Geometry: final body of the model. Coordinates: model frame, mm. Face numbers are marked on the shaded views. A direction names the side the tool comes from. Round coordinates to 2 decimals unless told otherwise and drop trailing zeros. Write each loop counter-clockwise with the first axis right and the second up, starting at its lowest first coordinate (ties: lowest second). Pieces come first, ordered by that corner, then holes. Notation, with made-up numbers: M -28,-2.5 L 10,-2.5 A6 cw 10,4.5 Z; hole C 85.25,-19 d9. An arc over 180 degrees is marked long. Answer as CSV lines item,"result". Start each with the question number.
Q1. Section query C-C on x = 4. Output: boundary loops of the cut face in (y, z).
Q2. Section query D-D on z = -20. Output: boundary loops of the cut face in (x, y), and give its area (3 significant figures).
Q3. Ray query, probe 1 along Y at (x, z) = (4.5, 16); probe 2 along Z at (x, y) = (4.5, -11); probe 3 along Z at (x, y) = (5, -11). Return the intervals inside material, ascending.
Q4. Section query B-B on z = 4. Output: boundary loops of the cut face in (x, y), and give its area (3 significant figures).
Q5. First-contact query: pin 1 (2.5 mm diameter, centred on y = -11, z = 16, fed in from +X); pin 2 (12 mm diameter, centred on x = 36.5, y = 4, fed in from +Z); pin 3 (4 mm diameter, centred on x = 12.5, y = -2, fed in from -Z). Flat tips, straight axial feed; report the tip coordinate or a pass-through.
Q6. Mould query, pull axis X, two halves, no side actions, for the marked faces 4, 5 and 6. Classes: pulls with the +X half, pulls with the -X half, needs draft (parallel to the pull), parting line crosses it, or undercut.
Q7. Reachability of the marked faces 1, 2 and 3 from +Z, -Z, +X, -X, +Y, -Y: full face, straight path, thin tool, end or side. Return the list, or none.
Solid Edge part; units mm, degrees
sketch "Sketch1" plane through (0, 0, 0) normal (1, 0, 0) x (0, 1, 0)
  line L0 (-14.25, -27.25) -> (-14.25, 27.25)
  line L1 (-14.25, 27.25) -> (14.25, 27.25)
  line L2 (14.25, 27.25) -> (14.25, -27.25)
  line L3 (14.25, -27.25) -> (-14.25, -27.25)
extrude "Protrusion1" add sketch "Sketch1" along normal blind 7.7
sketch "Sketch2" plane through (7.7, 0, 0) normal (1, 0, 0) x (0, 1, 0)
  line L0 (14.25, 19.55) -> (-14.25, 19.55)
  line L1 (-14.25, 19.55) -> (-14.25, 27.25)
  line L2 (-14.25, 27.25) -> (14.25, 27.25)
  line L3 (14.25, 27.25) -> (14.25, 19.55)
extrude "Extrusionsausprägung_2" add sketch "Sketch2" along normal blind 14.11
hole "Bohrung_1" at (0, 11, -24) direction (1, 0, 0) diameter 3.1 end through all
pattern_linear "Pattern1" count 2 spacing 22 along (0, -1, 0) count 2 spacing 40 along (0, 0, 1) of "Bohrung_1"
draft "Formschräge_3" angle 45 neutral plane through (18.75, 0, 19.55) normal (0, 0, -1) pull direction (0, 0, -1) face at (21.81, 9.215, 26.0437)
sketch "Sketch3" plane through (29.505, 0, 27.245) normal (0.7071068, 0, -0.7071068) x (0, 1, 0)
  line L0 (-14.25, -10.8824) -> (14.25, -10.8824)
  line L1 (14.25, -10.8824) -> (14.25, -3.1824)
  line L2 (14.25, -3.1824) -> (-14.25, -3.1824)
  line L3 (-14.25, -3.1824) -> (-14.25, -10.8824)
extrude "Extrusionsausprägung_3" add sketch "Sketch3" along normal blind 23
sketch "Sketch4" plane through (32.5061, -14.25, 0) normal (0, -1, 0) x (1, 0, 0)
  line L0 (-5.2514, 24.9947) -> (-7.5067, 27.25)
extrude "Cutout1" cut sketch "Sketch4" against normal through all material side at (26.1624, -14.25, 26.1577)
hole "Bohrung_10" at (31.123, -9.25, 10.237) direction (0.7071068, 0, 0.7071068) diameter 3.2 end up to next
hole "Hole1" at (31.123, 9.25, 10.237) direction (0.7071068, 0, 0.7071068) diameter 3.2 end up to next
sketch "Sketch5" plane through (28.8811, 0, 12.4789) normal (-0.7071068, 0, -0.7071068) x (0.7071068, 0, -0.7071068)
  line L0 (4.7872, 12.05) -> (1.554, 12.05)
  line L1 (1.554, 12.05) -> (-0.0626, 9.25)
  line L2 (-0.0626, 9.25) -> (1.554, 6.45)
  line L3 (1.554, 6.45) -> (4.7872, 6.45)
  line L4 (4.7872, 6.45) -> (6.4038, 9.25)
  line L5 (6.4038, 9.25) -> (4.7872, 12.05)
extrude "Extrusionsausschnitt_2" cut sketch "Sketch5" against normal blind 3
sketch "Sketch6" plane through (28.8811, 0, 12.4789) normal (-0.7071068, 0, -0.7071068) x (0.7071068, 0, -0.7071068)
  line L0 (4.7872, -12.05) -> (6.4038, -9.25)
  line L1 (6.4038, -9.25) -> (4.7872, -6.45)
  line L2 (4.7872, -6.45) -> (1.554, -6.45)
  line L3 (1.554, -6.45) -> (-0.0626, -9.25)
  line L4 (-0.0626, -9.25) -> (1.554, -12.05)
  line L5 (1.554, -12.05) -> (4.7872, -12.05)
extrude "Extrusionsausschnitt_3" cut sketch "Sketch6" against normal blind 3
sketch "Sketch7" plane through (0, 0, 0) normal (0, -1, 0) x (1, 0, 0)
  line L0 (7.7, -27.25) -> (18.3066, -37.8566)
  line L1 (18.3066, -37.8566) -> (12.8619, -43.3013)
  line L2 (12.8619, -43.3013) -> (0, -30.4394)
  line L3 (0, -30.4394) -> (0, -27.25)
  line L4 (0, -27.25) -> (7.7, -27.25)
extrude "Extrusionsausprägung_14" add sketch "Sketch7" along normal mid plane 28.5
sketch "Sketch8" plane through (13.0033, 0, -32.5533) normal (0.7071068, 0, 0.7071068) x (0.7071068, 0, -0.7071068)
  line L0 (3, 5.0179) -> (3, 8.4821)
  line L1 (3, 8.4821) -> (0, 10.2141)
  line L2 (0, 10.2141) -> (-3, 8.4821)
  line L3 (-3, 8.4821) -> (-3, 5.0179)
  line L4 (-3, 5.0179) -> (0, 3.2859)
  line L5 (0, 3.2859) -> (3, 5.0179)
  line L6 (3, -8.4821) -> (3, -5.0179)
  line L7 (3, -5.0179) -> (0, -3.2859)
  line L8 (0, -3.2859) -> (-3, -5.0179)
  line L9 (-3, -5.0179) -> (-3, -8.4821)
  line L10 (-3, -8.4821) -> (0, -10.2141)
  line L11 (0, -10.2141) -> (3, -8.4821)
extrude "Extrusionsausschnitt_6" cut sketch "Sketch8" against normal blind 3
hole "Bohrung_12" at (13.0033, 6.75, -32.5533) direction (-0.7071068, 0, -0.7071068) diameter 3.2 end up to next
hole "Hole2" at (13.0033, -6.75, -32.5533) direction (-0.7071068, 0, -0.7071068) diameter 3.2 end up to next
hole "Hole3" [suppressed]
hole "Hole4" [suppressed]
properties material "Finger_Unterbau"
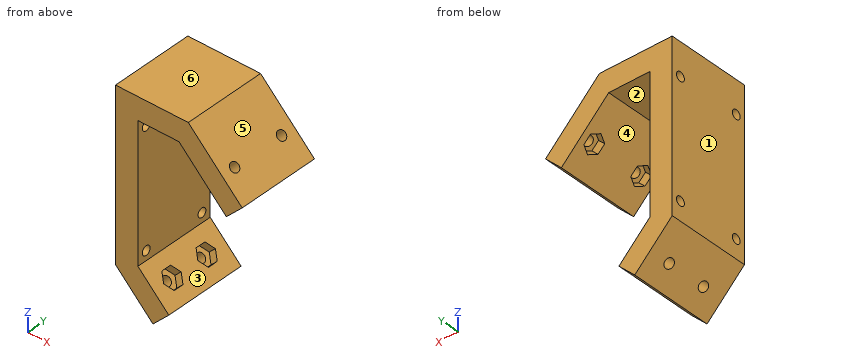
Entries:
1,outline,"M -14.25,-34.44 L 14.25,-34.44 L 14.25,27.25 L -14.25,27.25 Z; hole C -11,-24 d3.1; hole C -11,16 d3.1; hole C 11,-24 d3.1; hole C 11,16 d3.1"
2,outline,"M 0,-14.25 L 7.7,-14.25 L 7.7,14.25 L 0,14.25 Z"
2,area,"219 mm^2"
3,probe 1,"y = -14.25 to -12.55, -9.45 to 9.45, 12.55 to 14.25"
3,probe 2,"z = -34.94 to -25.55, -22.45 to 14.45, 17.55 to 27.25"
3,probe 3,"z = -35.44 to -25.55, -22.45 to 14.45, 17.55 to 27.25"
4,outline,"M 0,-14.25 L 7.7,-14.25 L 7.7,14.25 L 0,14.25 Z; M 37.36,-14.25 L 38.79,-14.25 L 38.79,14.25 L 37.36,14.25 Z"
4,area,"260 mm^2"
5,pin 1,"stops at x = 37.5"
5,pin 2,"stops at z = 21.75"
5,pin 3,"stops at z = -43.3"
6,face 4,"undercut"
6,face 5,"pulls with the +X half"
6,face 6,"needs draft"
7,face 1,"+Z, -Z, -X, +Y, -Y"
7,face 2,"+Y, -Y"
7,face 3,"+X, +Y, -Y"
